Part model, mm, in its own coordinate system. A direction names the side the tool comes from. Give positions to 0.01 mm unless a question says otherwise; leave off trailing zeros. Write each loop counter-clockwise with the first axis right and the second up, starting at its lowest first coordinate (ties: lowest second). Pieces come first, ordered by that corner, then holes. Notation, with made-up numbers: M -8,6 L 51,6 A20 ccw 51,38 Z; hole C 32.25,-23 d4. An arc over 180 degrees is marked long. Use a Markdown table: item, result. Add a question column.
from build123d import *

# Parameters (mm, degrees)
F0_R     = 5
F1_DEPTH = 7
F4_R     = 5.5
F4_R_2   = 5
F5_DEPTH = 2
F7_DEPTH = 28
F8_DEPTH = 26


with BuildPart() as f1:
    # F0 (on Top) → F1 (new body)
    with BuildSketch(Plane.XY):
        Circle(F0_R)
    extrude(amount=F1_DEPTH)

    # F2 (on Front) → F3 (revolve)
    with BuildSketch(Plane.XZ):
        with BuildLine():
            Line((0, 12), (0, 7))
            Line((0, 7), (5, 7))
            ThreePointArc((5, 7), (3.5355339059, 10.5355339059), (0, 12))
        make_face()
    revolve(axis=Axis((0, 0, 10.5024230517), (0, 0, -1)))

    # F4 (on face) → F5 (join)
    with BuildSketch(Plane(origin=(0, 0, 0), x_dir=(1, 0, 0), z_dir=(0, 0, -1))):
        Circle(F4_R)
        Circle(F4_R_2, mode=Mode.SUBTRACT)
        Circle(F4_R_2)
    extrude(amount=F5_DEPTH)

    # F6 (on face) → F7 (join)
    with BuildSketch(Plane(origin=(0, 0, -2), x_dir=(1, 0, 0), z_dir=(0, 0, -1))):
        Polygon((-1, -0.3), (-1, 0), (-1, 0.3), (-1.5, 0.3), (-1.5, -0.3), align=None)
    extrude(amount=F7_DEPTH)

    # F6 (on face) → F8 (join)
    with BuildSketch(Plane(origin=(0, 0, -2), x_dir=(1, 0, 0), z_dir=(0, 0, -1))):
        Polygon((1, 0.3), (1, 0), (1, -0.3), (1.5, -0.3), (1.5, 0.3), align=None)
    extrude(amount=F8_DEPTH)


solid = f1.part
1. Cut at B-B (x = 0). Write the cut outline in (y, z).
2. Tool access for faces 1 (the cylindrical face through (-1.19, 5.37, -0.99)), 2 (the flat face through (1.6, 4.9, 0)): list every direction of +Z, -Z, +X, -X, +Y, -Y with a clear straight run to the whole face (end or side of a thin tool).
3. Flat gauge pins, fed straight in: pin 1 (5 mm diameter, centred on x = -1.5, z = -8, fed in from +Y); pin 2 (0.5 mm diameter, centred on y = 0, z = -16.5, fed in from -X); pin 3 (0.7 mm diameter, centred on y = 0, z = -13.5, fed in from +X). Where does each tip first touch, or does it go through?
4. Cut at C-C (y = -3). Write the cut outline in (x, z), then the cut area to 3 significant figures.
5. Drill centre lines: probe 1 along X at (y, z) = (0, -7.5); probe 2 along Z at (x, y) = (1, 5); probe 3 along Z at (x, y) = (2.5, -3). Where is each one in solid material? Low to high. Write a range as [from, to].
6. Cut at A-A (z = -12). Write the cut outline in (x, y), then the cut area to 3 significant figures.
A:
| question | item | result |
|---|---|---|
| 1 | outline | M -5.5,-2 L 5.5,-2 L 5.5,0 L 5,0 L 5,7 A5 ccw -5,7 L -5,0 L -5.5,0 Z |
| 2 | face 1 | +Z, -Z |
| 2 | face 2 | +Z |
| 3 | pin 1 | stops at y = 0.3 |
| 3 | pin 2 | stops at x = -1.5 |
| 3 | pin 3 | stops at x = 1.5 |
| 4 | outline | M -4.61,-2 L 4.61,-2 L 4.61,0 L 4,0 L 4,7 A4 ccw -4,7 L -4,0 L -4.61,0 Z |
| 4 | area | 99.6 mm² |
| 5 | probe 1 | x = [-1.5, -1], [1, 1.5] |
| 5 | probe 2 | z = [-2, 0] |
| 5 | probe 3 | z = [-2, 10.12] |
| 6 | outline | M -1.5,-0.3 L -1,-0.3 L -1,0.3 L -1.5,0.3 Z; M 1,-0.3 L 1.5,-0.3 L 1.5,0.3 L 1,0.3 Z |
| 6 | area | 0.600 mm² |
